from build123d import *

# Parameters (mm, degrees)
F0_W      = 101.6
F0_H      = 101.6
F1_DEPTH  = 3.175
F5_DEPTH  = 50.8
F6_DEPTH  = 57.15
F7_DEPTH  = 63.5
F8_DEPTH  = 69.85
F9_DEPTH  = 76.2
F10_DEPTH = 69.85
F11_DEPTH = 63.5
F12_DEPTH = 57.15
F13_DEPTH = 50.8
F14_W     = 126.8053464592
F14_H     = 131.9155991077
F14_W_2   = 101.6
F14_H_2   = 101.6
F15_DEPTH = 12.7


with BuildPart() as f1:
    # F0 (on Top) → F1 (new body)
    with BuildSketch(Plane.XY):
        Rectangle(F0_W, F0_H)
    extrude(amount=F1_DEPTH)

    # F4 (on line) → F5 (join, symmetric)
    with BuildSketch(Plane(origin=(0, 0, 0), x_dir=(-0.7071067812, 0.7071067812, 0), z_dir=(0.7071067812, 0.7071067812, 0))):
        with BuildLine():
            Line((26.9160220652, 3.175), (26.9160220652, 4.7411556013))
            ThreePointArc((26.9160220652, 4.7411556013), (26.9160579383, 4.7518278006), (26.9160220652, 4.7625))
            ThreePointArc((26.9160220652, 4.7625), (25.3232218085, 6.3393188323), (23.7410579383, 4.7518278006))
            Line((23.7410579383, 4.7518278006), (23.7410579383, 3.175))
            Line((23.7410579383, 3.175), (26.9160220652, 3.175))
        make_face()
    extrude(amount=F5_DEPTH, both=True)

    # F4 (on line) → F6 (join, symmetric)
    with BuildSketch(Plane(origin=(0, 0, 0), x_dir=(-0.7071067812, 0.7071067812, 0), z_dir=(0.7071067812, 0.7071067812, 0))):
        with BuildLine():
            ThreePointArc((20.5660220652, 4.7625), (18.9732218085, 6.3393188323), (17.3910579383, 4.7518278006))
            Line((17.3910579383, 4.7518278006), (17.3910579383, 3.175))
            Line((17.3910579383, 3.175), (20.5660220652, 3.175))
            Line((20.5660220652, 3.175), (20.5660220652, 4.7411556013))
            Line((20.5660220652, 4.7411556013), (20.5660220652, 4.7625))
        make_face()
    extrude(amount=F6_DEPTH, both=True)

    # F4 (on line) → F7 (join, symmetric)
    with BuildSketch(Plane(origin=(0, 0, 0), x_dir=(-0.7071067812, 0.7071067812, 0), z_dir=(0.7071067812, 0.7071067812, 0))):
        with BuildLine():
            ThreePointArc((14.2160220652, 4.7625), (12.6232218085, 6.3393188323), (11.0410579383, 4.7518278006))
            Line((11.0410579383, 4.7518278006), (11.0410579383, 3.175))
            Line((11.0410579383, 3.175), (14.2160220652, 3.175))
            Line((14.2160220652, 3.175), (14.2160220652, 4.7411556013))
            Line((14.2160220652, 4.7411556013), (14.2160220652, 4.7625))
        make_face()
    extrude(amount=F7_DEPTH, both=True)

    # F4 (on line) → F8 (join, symmetric)
    with BuildSketch(Plane(origin=(0, 0, 0), x_dir=(-0.7071067812, 0.7071067812, 0), z_dir=(0.7071067812, 0.7071067812, 0))):
        with BuildLine():
            ThreePointArc((7.8660220652, 4.7625), (6.2732218085, 6.3393188323), (4.6910579383, 4.7518278006))
            Line((4.6910579383, 4.7518278006), (4.6910579383, 3.175))
            Line((4.6910579383, 3.175), (7.8660220652, 3.175))
            Line((7.8660220652, 3.175), (7.8660220652, 4.7411556013))
            Line((7.8660220652, 4.7411556013), (7.8660220652, 4.7625))
        make_face()
    extrude(amount=F8_DEPTH, both=True)

    # F4 (on line) → F9 (join, symmetric)
    with BuildSketch(Plane(origin=(0, 0, 0), x_dir=(-0.7071067812, 0.7071067812, 0), z_dir=(0.7071067812, 0.7071067812, 0))):
        with BuildLine():
            ThreePointArc((1.5160220652, 4.7625), (-0.0767781915, 6.3393188323), (-1.6589420617, 4.7518278006))
            Line((-1.6589420617, 4.7518278006), (-1.6589420617, 3.175))
            Line((-1.6589420617, 3.175), (1.5160220652, 3.175))
            Line((1.5160220652, 3.175), (1.5160220652, 4.7411556013))
            Line((1.5160220652, 4.7411556013), (1.5160220652, 4.7625))
        make_face()
    extrude(amount=F9_DEPTH, both=True)

    # F4 (on line) → F10 (join, symmetric)
    with BuildSketch(Plane(origin=(0, 0, 0), x_dir=(-0.7071067812, 0.7071067812, 0), z_dir=(0.7071067812, 0.7071067812, 0))):
        with BuildLine():
            ThreePointArc((-4.8339779348, 4.7625), (-6.4267781915, 6.3393188323), (-8.0089420617, 4.7518278006))
            Line((-8.0089420617, 4.7518278006), (-8.0089420617, 3.175))
            Line((-8.0089420617, 3.175), (-4.8339779348, 3.175))
            Line((-4.8339779348, 3.175), (-4.8339779348, 4.7411556013))
            Line((-4.8339779348, 4.7411556013), (-4.8339779348, 4.7625))
        make_face()
    extrude(amount=F10_DEPTH, both=True)

    # F4 (on line) → F11 (join, symmetric)
    with BuildSketch(Plane(origin=(0, 0, 0), x_dir=(-0.7071067812, 0.7071067812, 0), z_dir=(0.7071067812, 0.7071067812, 0))):
        with BuildLine():
            ThreePointArc((-11.1839779348, 4.7625), (-12.7767781915, 6.3393188323), (-14.3589420617, 4.7518278006))
            Line((-14.3589420617, 4.7518278006), (-14.3589420617, 3.175))
            Line((-14.3589420617, 3.175), (-11.1839779348, 3.175))
            Line((-11.1839779348, 3.175), (-11.1839779348, 4.7411556013))
            Line((-11.1839779348, 4.7411556013), (-11.1839779348, 4.7625))
        make_face()
    extrude(amount=F11_DEPTH, both=True)

    # F4 (on line) → F12 (join, symmetric)
    with BuildSketch(Plane(origin=(0, 0, 0), x_dir=(-0.7071067812, 0.7071067812, 0), z_dir=(0.7071067812, 0.7071067812, 0))):
        with BuildLine():
            ThreePointArc((-17.5339779348, 4.7625), (-19.1267781915, 6.3393188323), (-20.7089420617, 4.7518278006))
            Line((-20.7089420617, 4.7518278006), (-20.7089420617, 3.175))
            Line((-20.7089420617, 3.175), (-17.5339779348, 3.175))
            Line((-17.5339779348, 3.175), (-17.5339779348, 4.7411556013))
            Line((-17.5339779348, 4.7411556013), (-17.5339779348, 4.7625))
        make_face()
    extrude(amount=F12_DEPTH, both=True)

    # F4 (on line) → F13 (join, symmetric)
    with BuildSketch(Plane(origin=(0, 0, 0), x_dir=(-0.7071067812, 0.7071067812, 0), z_dir=(0.7071067812, 0.7071067812, 0))):
        with BuildLine():
            ThreePointArc((-23.8839779348, 4.7625), (-25.4767781915, 6.3393188323), (-27.0589420617, 4.7518278006))
            Line((-27.0589420617, 4.7518278006), (-27.0589420617, 3.175))
            Line((-27.0589420617, 3.175), (-23.8839779348, 3.175))
            Line((-23.8839779348, 3.175), (-23.8839779348, 4.7411556013))
            Line((-23.8839779348, 4.7411556013), (-23.8839779348, 4.7625))
        make_face()
    extrude(amount=F13_DEPTH, both=True)

    # F14 (on Top) → F15 (cut)
    with BuildSketch(Plane.XY):
        with Locations((0.9669456631, -0.0485852361)):
            Rectangle(F14_W, F14_H)
        Rectangle(F14_W_2, F14_H_2, mode=Mode.SUBTRACT)
    extrude(amount=F15_DEPTH, mode=Mode.SUBTRACT)


solid = f1.part
Design review of the part built by this model. Coordinates are the model's own, in mm. A direction names the side the tool comes from. Round coordinates to 2 decimals unless told otherwise and drop trailing zeros. Use a Markdown table: item, result. Add a question column.
1. Clearance check with a flat-ended pin moving along its axis: pin 1 (10 mm diameter, centred on x = 34.5, y = -20.5, fed in from +Z) (3 decimals). State where the tip first meets the part, or that it passes through.
2. For faces 1 (the face through (-18.588, 19.477, 3.947)), 2 (the face through (5, -1, 3.175)), 3 (the face through (-1, -50.8, 2)), 4 (the face through (33, -33, 3.175)), list the 3-axis set-ups (+Z, -Z, +X, -X, +Y, -Y) from which the entire face can be reached by the end or side of a thin tool; tool diameter is ignored.
3. Wall thickness on probe 1 along Y at (x, z) = (-45, 4) (1 decimal); probe 2 along X at (y, z) = (36, 5.75); probe 3 along X at (y, z) = (44.5, 5): over which ranges is each line inside the solid? List them lowest first.
4. Mouldability with a two-part tool opening along Y and no side actions: class faces 5 (the face through (-1, 1, 0)), 6 (the face through (-1, 50.8, 2)), 7 (the face through (19.577, -18.69, 3.974)), 8 (the face through (17.363, -16.414, 3.958)) as +Y half, -Y half, draft (parallel to the pull), parting line (faces both ways), or undercut.
Output:
| question | item | result |
|---|---|---|
| 1 | pin 1 | stops at z = 3.175 |
| 2 | face 1 | +Z, -X, +Y |
| 2 | face 2 | +Z |
| 2 | face 3 | +Z, -Z, +X, -X, -Y |
| 2 | face 4 | +Z, +X, -Y |
| 3 | probe 1 | y = -47.3 to -42.9, -38.4 to -33.9, -29.4 to -24.9, -20.4 to -15.9, -11.4 to -6.9 |
| 3 | probe 2 | x = -1.57 to 1.93, 7.41 to 10.91, 16.39 to 19.89, 25.38 to 28.87, 34.36 to 37.85, 43.34 to 46.83 |
| 3 | probe 3 | x = 6.46 to 10.9, 15.44 to 19.88, 24.42 to 28.86, 33.4 to 37.84, 42.38 to 46.82 |
| 4 | face 5 | draft |
| 4 | face 6 | +Y half |
| 4 | face 7 | -Y half |
| 4 | face 8 | undercut |
